Here's how the part is built. I have some questions about the finished solid (model axes, mm). Face numbers are marked on the shaded views. A direction names the side the tool comes from. Coordinates: 2 decimals unless noted, no trailing zeros. Write each loop counter-clockwise with the first axis right and the second up, starting at its lowest first coordinate (ties: lowest second). Pieces come first, ordered by that corner, then holes.
Item 1: I want a section at C-C (z = -0.75). Count the separate pieces of the cut face and the enclosed holes in it, and give its area (3 significant figures).
Item 2: I want a section at D-D (y = 16). Please give me the cut outline in (x, z), and give its area (3 significant figures).
Item 3: Please list where these lines run through material, in increasing order: line 1 (X direction, y = 9, z = 0); line 2 (Y direction, x = 12.5, z = 3); line 3 (Y direction, x = 17, z = -6).
Item 4: I want a section at B-B (x = 12.5). Please give me the cut outline in (y, z).
Item 5: I want a section at A-A (y = 4). Please give me the cut outline in (x, z).
Item 6: I'm going to push flat-ended pins straight in: P1, Ø2, axis at x = 16, z = -5, coming from the +Y side; P2, Ø7, axis at x = 0, z = 0, coming from the +Y side; P3, Ø5, axis at x = 25, z = 0, coming from the +Y side; P4, Ø6, axis at y = 18, z = 5, coming from the +X side. Where does each tip first touch, or does it pass through?
Item 7: For the marked faces 3 and 4, which set-ups out of +Z, -Z, +X, -X, +Y, -Y let a thin tool reach every point of the face, with its end or its side?
Item 8: If we mould it in two halves opening along X, with no side actions, what happens to the marked faces 1 and 2? For each: pulls with the +X half, pulls with the -X half, needs draft (parallel to the pull), parting line crosses it, or undercut.
Autodesk Inventor part; units mm, degrees
ref_plane "Work Plane1" through (12.5, 0, 0) normal (1, 0, 0) x (0, 1, 0)
ref_plane "XZ Plane" through (0, 0, 0) normal (0, 1, 0) x (-1, 0, 0)
ref_plane "XY Plane" through (0, 0, 0) normal (0, 0, 1) x (1, 0, 0)
sketch "Sketch1" plane through (0, 0, 0) normal (0, 1, 0) x (-1, 0, 0)
  circle A0 centre (0, 0) radius 7.5
  circle A1 centre (0, 0) radius 3
  dimension "d0" = 15
  dimension "d1" = 6
extrude "Extrusion1" add sketch "Sketch1" along normal blind 25
sketch "Sketch2" plane through (0, 25, 0) normal (0, 1, 0) x (1, 0, 0)
  circle A0 centre (0, 0) radius 3
  circle A1 centre (0, 0) radius 2.75
  circle A2 centre (0, 0) radius 4
  dimension "d4" = 5.5
  dimension "d5" = 8
extrude "Extrusion2" add sketch "Sketch2" along normal blind 7 contours A2
fillet "Fillet1" radius 6 1 edges at (-4, 25, 0)
fillet "Fillet2" radius 6 2 edges at (0, 25, -7.5) (0, 25, 7.5)
ref_plane "Work Plane1" through (12.5, 0, 0) normal (1, 0, 0) x (0, 1, 0)
mirror "Mirror1" about plane through (12.5, 0, 0) normal (1, 0, 0) of "Extrusion1", "Extrusion2", "Fillet1", "Fillet2"
sketch "Sketch3" plane through (0, 0, 0) normal (0, 1, 0) x (-1, 0, 0)
  circle A0 centre (-25, 0) radius 3
  line L0 (-25, 0) -> (-25, 3)
  line L1 (-25, 0) -> (-25, -3)
  line L2 (0, 0) -> (0, -3)
  circle A1 centre (0, 0) radius 3
  line L3 (0, 0) -> (0, 3)
  line L4 (-25, 3) -> (0, 3)
  line L5 (0, 3) -> (0, 7.5)
  line L6 (0, 7.5) -> (-25, 7.5)
  line L7 (-25, 7.5) -> (-25, 3)
  line L8 (-25, -3) -> (0, -3)
  line L9 (0, -3) -> (0, -7.5)
  line L10 (0, -7.5) -> (-25, -7.5)
  line L11 (-25, -7.5) -> (-25, -3)
  point P0 (0, -3)
  point P1 (0, 3)
  dimension "d11" = 25
  dimension "d12" = 4.5
  dimension "d13" = 25
  dimension "d14" = 4.5
extrude "Extrusion3" add sketch "Sketch3" along normal blind 20 contours A0 L4 A1 L8 | L7 L6 L5 L4 | L8 L9 L10 L11
sketch "Sketch4" plane through (0, 0, 7.5) normal (0, 0, 1) x (1, 0, 0)
  line L0 (25, 20) -> (0, 20)
  circle A0 centre (12.5, 5) radius 3
  line L1 (0, 0) -> (25, 0)
  line L2 (0, 0) -> (0, 20)
  point P0 (25, 15)
  point P1 (0, 15)
  dimension "d18" = 6
  dimension "d21" = 5
  dimension "d22" = 12.5
extrude "Extrusion4" cut sketch "Sketch4" against normal through all
properties part number "4mm_Roller_Spacer_full"
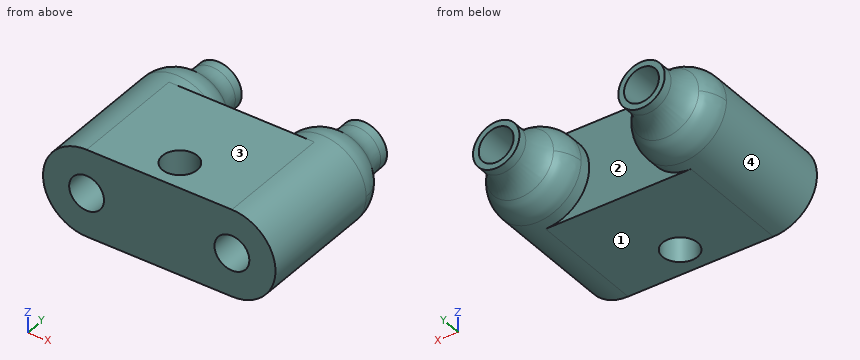
Answer:
1. separate pieces: 3
1. enclosed holes: 1
1. area: 675 mm2
2. outline: (0, -7.5) - (25, -7.5) arc R7.5 ccw to (25, 7.5) - (0, 7.5) arc R7.5 ccw to start; hole circle Ø6 at (0, 0); hole circle Ø6 at (25, 0)
2. area: 495 mm2
3. line 1: x = -7.5 to -3, 3 to 22, 28 to 32.5
3. line 2: y = 0 to 2, 8 to 20
3. line 3: y = 0 to 20
4. outline: (0, -7.5) - (2, -7.5) - (2, 7.5) - (0, 7.5) - close; (8, -7.5) - (20, -7.5) - (20, 7.5) - (8, 7.5) - close
5. outline: (0, -7.5) - (9.67, -7.5) - (9.67, 7.5) - (0, 7.5) arc R7.5 ccw to start; (15.33, -7.5) - (25, -7.5) arc R7.5 ccw to (25, 7.5) - (15.33, 7.5) - close; hole circle Ø6 at (0, 0); hole circle Ø6 at (25, 0)
6. P1: stops at y = 20
6. P2: stops at y = 32
6. P3: passes through
6. P4: stops at x = 32.23
7. face 3: +Z, +X, -X, +Y, -Y
7. face 4: +Y
8. face 1: needs draft
8. face 2: undercut
